Autodesk Inventor part; units mm, degrees
ref_plane "YZ Plane" through (0, 0, 0) normal (1, 0, 0) x (0, 1, 0)
ref_plane "XZ Plane" through (0, 0, 0) normal (0, 1, 0) x (-1, 0, 0)
ref_plane "XY Plane" through (0, 0, 0) normal (0, 0, 1) x (1, 0, 0)
sketch "스케치1" plane through (0, 0, 0) normal (0, 1, 0) x (-1, 0, 0)
  line L0 (20.5, 10) -> (-20.5, 10)
  line L1 (-22.5, 8) -> (-22.5, -8)
  line L2 (-20.5, -10) -> (20.5, -10)
  line L3 (22.5, -8) -> (22.5, 8)
  line L4 (22.5, 10) -> (-22.5, -10) construction
  line L5 (-22.5, 10) -> (22.5, -10) construction
  line L6 (20.5, 8.25) -> (-20.5, 8.25)
  line L7 (-20.5, 8.25) -> (-20.5, -8.25)
  line L8 (-20.5, -8.25) -> (20.5, -8.25)
  line L9 (20.5, -8.25) -> (20.5, 8.25)
  line L10 (20.5, 8.25) -> (-20.5, -8.25) construction
  line L11 (-20.5, 8.25) -> (20.5, -8.25) construction
  circle A0 centre (20.5, -8.25) radius 1.1
  circle A1 centre (-20.5, -8.25) radius 1.1
  circle A2 centre (-20.5, 8.25) radius 1.1
  circle A3 centre (20.5, 8.25) radius 1.1
  arc A4 (20.5, -10) -> (22.5, -8) centre (20.5, -8) ccw
  arc A5 (22.5, 8) -> (20.5, 10) centre (20.5, 8) ccw
  arc A6 (-20.5, 10) -> (-22.5, 8) centre (-20.5, 8) ccw
  arc A7 (-22.5, -8) -> (-20.5, -10) centre (-20.5, -8) ccw
  line L12 (-22.5, 10) -> (22.5, 10)
  line L13 (22.5, 10) -> (22.5, -10)
  line L14 (22.5, -10) -> (-22.5, -10)
  line L15 (-22.5, -10) -> (-22.5, 10)
  line L16 (-22.5, 10) -> (22.5, -10) construction
  line L17 (22.5, 10) -> (-22.5, -10) construction
  point P0 (0, 0)
  dimension "d0" = 45
  dimension "d1" = 20
  dimension "d2" = 41
  dimension "d3" = 16.5
  dimension "d4" = 2.2
  dimension "d5" = 2.2
  dimension "d6" = 2.2
  dimension "d7" = 2.2
  dimension "d8" = 2
extrude "돌출1" add sketch "스케치1" along normal blind 3 contours A5 L3 A4 L2 A7 L1 A6 L0 | L12 L13 A5 | A6 L15 L12 | L13 L14 A4 | A7 L14 L15 | L6 A3 L9 A0 L8 A1 L7 A2
sketch "스케치6" plane through (-22.5, 0, 10) normal (0, 0, 1) x (1, 0, 0)
  line L0 (45, 3) -> (0, 3)
  line L1 (12.5, 0) -> (32.5, 0)
  line L2 (32.5, 0) -> (32.5, 3)
  line L3 (32.5, 3) -> (12.5, 3)
  line L4 (12.5, 3) -> (12.5, 0)
  line L5 (12.5, 0) -> (32.5, 3) construction
  line L6 (32.5, 0) -> (12.5, 3) construction
  point P0 (22.5, 0)
  point P1 (22.5, 1.5)
  dimension "d23" = 20
extrude "돌출5" add sketch "스케치6" along normal blind 8
sketch "스케치7" plane through (0, 0, 0) normal (0, -1, 0) x (1, 0, 0)
  line L0 (-10, 18) -> (10, 18)
  line L1 (-10, 10) -> (-10, 18)
  line L2 (10, 18) -> (-10, 18)
  line L3 (-10, 18) -> (-10, 15)
  line L4 (-10, 15) -> (10, 15)
  line L5 (10, 15) -> (10, 18)
  point P0 (0, 0)
  dimension "d26" = 3
extrude "돌출6" add sketch "스케치7" along normal blind 100
sketch "스케치8" plane through (10, 0, 15) normal (0, 0, -1) x (-1, 0, 0)
  line L0 (20, -100) -> (0, -100)
  line L1 (10, -100) -> (10, -90)
  line L2 (10, -90) -> (10, -40)
  circle A0 centre (10, -40) radius 3.15
  circle A1 centre (10, -90) radius 3.15
  point P0 (10, 0)
  dimension "d29" = 10
  dimension "d30" = 50
  dimension "d31" = 6.3
  dimension "d32" = 6.3
extrude "돌출7" cut sketch "스케치8" against normal blind 100
sketch "스케치9" plane through (0, 3, 0) normal (0, 1, 0) x (1, 0, 0)
  circle A0 centre (-20.5, 8.25) radius 1.1
  circle A1 centre (-20.5, 8.25) radius 1.1
  circle A2 centre (-20.5, 8.25) radius 1.6
  line L0 (22.5, 10) -> (-22.5, 10)
  line L1 (0, 10) -> (0, -18)
  line L2 (10, -18) -> (-10, -18)
  line L3 (-22.5, 10) -> (-22.5, -10)
  line L4 (-22.5, 0) -> (22.5, 0)
  line L5 (22.5, -10) -> (22.5, 10)
  circle A3 centre (20.5, 8.25) radius 1.1
  circle A4 centre (20.5, 8.25) radius 1.1
  circle A5 centre (20.5, 8.25) radius 1.6
  circle A6 centre (-20.5, -8.25) radius 1.1
  circle A7 centre (-20.5, -8.25) radius 1.1
  circle A8 centre (-20.5, -8.25) radius 1.6
  line L6 (22.5, -10) -> (-22.5, -10)
  circle A9 centre (20.5, -8.25) radius 1.1
  circle A10 centre (20.5, -8.25) radius 1.1
  circle A11 centre (20.5, -8.25) radius 1.6
  point P0 (0, 0)
  point P1 (0, -10)
  dimension "d35" = 0.5
extrude "돌출8" add sketch "스케치9" along normal blind 3 contours A2 | A5 | A8 | A11
sketch "스케치10" plane through (0, 3, 0) normal (0, 1, 0) x (1, 0, 0)
  line L0 (22.5, 10) -> (-22.5, 10)
  line L1 (0, 10) -> (-10, 10)
  line L2 (0, 10) -> (10, 10) construction
  line L3 (-10, 10) -> (10, 10)
  line L4 (10, 10) -> (10, 2)
  line L5 (10, 2) -> (-10, 2)
  line L6 (-10, 2) -> (-10, 10)
  point P0 (0, 0)
  dimension "d38" = 10
  dimension "d39" = 180
  dimension "d40" = 20
  dimension "d41" = 8
extrude "돌출9" cut sketch "스케치10" against normal blind 3
fillet "모깎기1" radius 5 2 edges at (-10, -100, 16.5) (10, -100, 16.5)
sketch "스케치11" plane through (-20.5, 6, -8.25) normal (0, 1, 0) x (1, 0, 0)
  circle A0 centre (0, 0) radius 1.1
  circle A1 centre (0, 0) radius 1.1
  circle A2 centre (0, -16.5) radius 1.1
  circle A3 centre (0, -16.5) radius 1.1
  circle A4 centre (41, 0) radius 1.1
  circle A5 centre (41, 0) radius 1.1
  circle A6 centre (41, -16.5) radius 1.1
  circle A7 centre (41, -16.5) radius 1.1
  point P0 (20.5, -8.25)
extrude "돌출10" add sketch "스케치11" against normal up to surface (6 mm away)
sketch "스케치12" plane through (20.5, 6, -8.25) normal (0, 1, 0) x (1, 0, 0)
  circle A0 centre (-41, 0) radius 1.6
  circle A1 centre (-41, 0) radius 0.4
  circle A2 centre (-41, -16.5) radius 1.6
  circle A3 centre (-41, -16.5) radius 0.4
  circle A4 centre (0, 0) radius 1.6
  circle A5 centre (0, 0) radius 0.4
  circle A6 centre (0, -16.5) radius 1.6
  circle A7 centre (0, -16.5) radius 0.4
  point P0 (-20.5, -8.25)
  dimension "d47" = 0.8
  dimension "d48" = 0.8
  dimension "d49" = 0.8
  dimension "d50" = 0.8
extrude "돌출11" add sketch "스케치12" along normal blind 3 contours A1 | A3 | A5 | A7
properties part number "sonic_sensor_holder"
Here's how the part is built. I have some questions about the finished solid (model axes, mm). A direction names the side the tool comes from. Coordinates: 2 decimals unless noted, no trailing zeros. Order: outer loops, then holes, each group sorted by start corner. A loop starts at its lowest first (then second) coordinate and runs counter-clockwise, first axis right, second up. Notation, with made-up numbers: (-34, 26) - (17, 26) arc R22 ccw to (17, 33) - close; hole circle Ø9 at (-39.5, -21.75). An arc over 180 degrees is marked (long way). One line per question, with ' | ' between items. Start each with the question number.
1. If we section it at A-A (y = -90): Write out the boundary of the cut face in (x, z).
2. If we section it at C-C (z = 1.5): Write out the boundary of the cut face in (x, y).
3. Please list where these lines run through material, in increasing order: line 1 along Y through (x, z) = (0, 16.95); line 2 along Y through (x, z) = (17.5, 1.75); line 3 along X through (y, z) = (-90, 15.95). Write a range as [from, to].
4. If we section it at B-B (x = 0): Write out the boundary of the cut face in (y, z).
5. If we section it at D-D (y = -57): Write out the boundary of the cut face in (x, z), and give its area (3 significant figures).
6. I'm going to push flat-ended pins straight in: pin 1 Ø4 at (y, z) = (-61, 14) entering from +X; pin 2 Ø3 at (x, z) = (-11, 6.5) entering from +Y; pin 3 Ø0.9 at (x, y) = (1.5, 1) entering from -Z. Where does each tip first touch, or does it pass through?
7. Which directions (+Z, -Z, +X, -X, +Y, -Y) give clear straight access to the entire face, cutting with the end or side of a thin tool? Please do faces 1 (the flat face through (21, 6, 9)), 2 (the flat face through (0, 0, 3)), 3 (the flat face through (-16, 1, 10)), 4 (the flat face through (-10, 2, -6)).
8. If we mould it in two halves opening along Z, with no side actions, what happens to faces 5 (the flat face through (0, -49, 15)), 6 (the flat face through (21, 6, -8)), 7 (the flat face through (0, -48, 18)), 8 (the flat face through (10, 2, -6))? For each: released by +Z, released by -Z, zero draft, split by the parting line, or undercut.
Model answer:
1) outline: (-10, 15) - (-3.15, 15) - (-3.15, 18) - (-10, 18) - close; (3.15, 15) - (10, 15) - (10, 18) - (3.15, 18) - close
2) outline: (-22.5, 0) - (22.5, 0) - (22.5, 3) - (-22.5, 3) - close
3) line 1: y = [-100, -93.15], [-86.85, -43.15], [-36.85, 3] | line 2: y = [0, 3] | line 3: x = [-10, -3.15], [3.15, 10]
4) outline: (-100, 15) - (-93.15, 15) - (-93.15, 18) - (-100, 18) - close; (-86.85, 15) - (-43.15, 15) - (-43.15, 18) - (-86.85, 18) - close; (-36.85, 15) - (0, 15) - (0, -2) - (3, -2) - (3, 18) - (-36.85, 18) - close
5) outline: (-10, 15) - (10, 15) - (10, 18) - (-10, 18) - close | area: 60.0 mm²
6) pin 1: stops at x = 10 | pin 2: stops at y = 3 | pin 3: stops at z = -2
7) face 1: +Y | face 2: -Z, +X, -X, -Y | face 3: +Z, -X, +Y, -Y | face 4: -Z, +Y, -Y
8) face 5: released by -Z | face 6: undercut | face 7: released by +Z | face 8: zero draft
